Geometry: final body of the model. Coordinates: model frame, mm. A direction names the side the tool comes from. Round coordinates to 2 decimals unless told otherwise and drop trailing zeros. Loops run counter-clockwise (first coordinate to the right, second up) from the corner with the lowest first, then second, coordinate; pieces in that order, holes last. Notation, with made-up numbers: (-20.75, -33.75) - (-9.75, -33.75) arc R25 ccw to (-9.75, -10.75) - close; hole circle Ø5 at (58.5, -36.5). An arc over 180 degrees is marked (long way). Answer as a JSON object with one key per item and string values. Group by question number.
Item 1: Section A-A (y = -12). Return the cut outline in (x, z).
Item 2: Reachability of faces 5 (the face through (12.7, 122.6, -0.7)), 6 (the face through (15, -19.577, -11)), 7 (the face through (9, 45, 4.362)), 8 (the face through (2.58, -37.76, -9.25)) from +Z, -Z, +X, -X, +Y, -Y: full face, straight path, thin tool, end or side. Return the list, or none.
Item 3: Section D-D (y = 53). Return the cut outline in (x, z).
Item 4: Line query: line 1 (X direction, y = -14.5, z = -4.75); line 2 (Z direction, x = 2.75, y = 59); line 3 (Y direction, x = 10.25, z = -0.25). Output: solid intervals per line, ascending.
Item 5: Section C-C (x = 7.5). Return the cut outline in (y, z).
Item 6: Section B-B (x = 1.5). Return the cut outline in (y, z), plus the area to 3 significant figures.
Item 7: Draft query along Z for faces 1 (the face through (15, -28, -14.688)), 2 (the face through (3, -34, -8.338)), 3 (the face through (15.28, -37.76, -9.25)), 4 (the face through (0, 45, -3)). Return one class per face: released by +Z, released by -Z, zero draft, split by the parting line, or undercut.
Item 8: First-contact query: pin 1 (1.5 mm diameter, centred on x = 16.5, z = -13, fed in from +Y); pin 2 (3 mm diameter, centred on x = 10.5, z = -3, fed in from -Y); pin 3 (5 mm diameter, centred on x = 11, z = -4, fed in from -Y); pin 4 (4 mm diameter, centred on y = -32.28, z = -1.99, fed in from +X). Flat tips, straight axial feed; report the tip coordinate or a pass-through.
```python
from build123d import *

# Parameters (mm, degrees)
F0_W      = 63.5
F0_H      = 12.7
F1_DEPTH  = 17.78
F2_W      = 5.08
F2_H      = 12.7
F3_DEPTH  = 25.4
F4_R      = 2.54
F5_DEPTH  = 25.4
F6_DEPTH  = 50.8
F7_DEPTH  = 76.2
F8_W      = 5.08
F8_H      = 12.7
F9_DEPTH  = 12.7
F11_W     = 5.08
F11_H     = 12.7
F12_DEPTH = 6.35
F13_DEPTH = 6.35
F15_DEPTH = 25.4
F10_R     = 2.54
F16_DEPTH = 25.4
F14_R     = 1.2823476499
F17_DEPTH = 25.4


# Not quite as in the source:
# - a feature names something its author has since deleted; it is built from what else it names


with BuildPart() as f1:
    # F0 (on Right) → F1 (new body)
    with BuildSketch(Plane.YZ):
        with Locations((10.0746992975, -1.9877629941)):
            Rectangle(F0_W, F0_H)
    extrude(amount=F1_DEPTH)

    # F2 (on face) → F3 (join)
    with BuildSketch(Plane.XZ.offset(21.6753007025)):
        with Locations((2.54, -1.9877629941)):
            Rectangle(F2_W, F2_H)
        with Locations((15.24, -1.9877629941)):
            Rectangle(F2_W, F2_H)
    extrude(amount=F3_DEPTH)

    # F4 (on face) → F5 (cut)
    with BuildSketch(Plane.YZ.offset(17.78)):
        with Locations((-32.2765819728, -1.9877629941)):
            Circle(F4_R)
        with BuildLine():
            ThreePointArc((-32.2765819728, -8.3377629941), (-38.3512132445, -1.9877629941), (-32.2765819728, 4.3622370059))
            Line((-32.2765819728, 4.3622370059), (-47.0753007025, 4.3622370059))
            Line((-47.0753007025, 4.3622370059), (-47.0753007025, -8.3377629941))
            Line((-47.0753007025, -8.3377629941), (-32.2765819728, -8.3377629941))
        make_face()
    extrude(amount=-F5_DEPTH, mode=Mode.SUBTRACT)

    # F6 (cut): a face of the model
    f6_faces = [f1.faces().sort_by_distance(p)[0] for p in [
        (8.89, -21.6753007025, -1.9877629941),
    ]]
    extrude(f6_faces, amount=-F6_DEPTH, mode=Mode.SUBTRACT)

    # F7 (add): a face of the model
    f7_faces = [f1.faces().sort_by_distance(p)[0] for p in [
        (8.89, 41.8246992975, -1.9877629941),
    ]]
    extrude(f7_faces, amount=F7_DEPTH)

    # F8 (on face) → F9 (join)
    with BuildSketch(Plane(origin=(0, 118.0246992975, 0), x_dir=(-1, 0, 0), z_dir=(0, 1, 0))):
        with Locations((-15.24, -1.9877629941)):
            Rectangle(F8_W, F8_H)
        with Locations((-2.54, -1.9877629941)):
            Rectangle(F8_W, F8_H)
    extrude(amount=F9_DEPTH)

    # F11 (on face) → F12 (join)
    with BuildSketch(Plane(origin=(0, 0, -8.3377629941), x_dir=(1, 0, 0), z_dir=(0, 0, -1))):
        with Locations((15.24, 25.9265819728)):
            Rectangle(F11_W, F11_H)
        with Locations((2.54, 25.9265819728)):
            Rectangle(F11_W, F11_H)
    extrude(amount=F12_DEPTH)

    # F13 (add): faces of the model
    f13_faces = [f1.faces().sort_by_distance(p)[0] for p in [
        (15.24, -32.2765819728, -11.5127629941),
        (2.54, -32.2765819728, -11.5127629941),
    ]]
    extrude(f13_faces, amount=F13_DEPTH)

    # F14 (on face) → F15 (cut)
    with BuildSketch(Plane.YZ.offset(17.78)):
        with BuildLine():
            ThreePointArc((-38.6265819728, -10.9001689166), (-37.7400292742, -9.2277758835), (-36.0694751143, -8.3377629941))
            Line((-36.0694751143, -8.3377629941), (-38.6265819728, -8.3377629941))
            Line((-38.6265819728, -8.3377629941), (-38.6265819728, -10.9001689166))
        make_face()
        with BuildLine():
            ThreePointArc((-36.0694751143, -14.6877629941), (-37.7400292742, -13.7977501047), (-38.6265819728, -12.1253570717))
            Line((-38.6265819728, -12.1253570717), (-38.6265819728, -14.6877629941))
            Line((-38.6265819728, -14.6877629941), (-36.0694751143, -14.6877629941))
        make_face()
    extrude(amount=-F15_DEPTH, mode=Mode.SUBTRACT)

    # F10 (on face) → F16 (cut)
    with BuildSketch(Plane.YZ.offset(17.78)):
        with BuildLine():
            ThreePointArc((125.2040266991, 4.3622370059), (130.0066745518, -1.9877629941), (125.2040266991, -8.3377629941))
            Line((125.2040266991, -8.3377629941), (130.7246992975, -8.3377629941))
            Line((130.7246992975, -8.3377629941), (130.7246992975, 4.3622370059))
            Line((130.7246992975, 4.3622370059), (125.2040266991, 4.3622370059))
        make_face()
        with Locations((125.2040266991, -1.9877629941)):
            Circle(F10_R)
    extrude(amount=-F16_DEPTH, mode=Mode.SUBTRACT)

    # F14 (on face) → F17 (cut)
    with BuildSketch(Plane.YZ.offset(17.78)):
        with Locations((-36.0694751144, -11.5127629941)):
            Circle(F14_R)
    extrude(amount=-F17_DEPTH, mode=Mode.SUBTRACT)


solid = f1.part
```
Values:
{
 "1": {"outline": "(0, -8.34) - (5.08, -8.34) - (5.08, 4.36) - (0, 4.36) - close; (12.7, -8.34) - (17.78, -8.34) - (17.78, 4.36) - (12.7, 4.36) - close"},
 "2": {"face 5": "+Z, -Z, +Y", "face 6": "-Z, +X, -X, +Y", "face 7": "+Z, +X, -X, +Y, -Y", "face 8": "+X, -X, -Y"},
 "3": {"outline": "(0, -8.34) - (17.78, -8.34) - (17.78, 4.36) - (0, 4.36) - close"},
 "4": {"line 1": "x = 0 to 5.08, 12.7 to 17.78", "line 2": "z = -8.34 to 4.36", "line 3": "y = 29.12 to 118.02"},
 "5": {"outline": "(29.12, -8.34) - (118.02, -8.34) - (118.02, 4.36) - (29.12, 4.36) - close"},
 "6": {"outline": "(-38.63, -12.13) arc R3.23 ccw to (-36.07, -14.69) - (-19.58, -14.69) - (-19.58, -8.34) - (125.2, -8.34) arc R6.6 ccw to (125.2, 4.36) - (-32.28, 4.36) arc R6.36 ccw to (-32.28, -8.34) - (-36.07, -8.34) arc R3.23 ccw to (-38.63, -10.9) - close; hole circle Ø2.56 at (-36.07, -11.51); hole circle Ø5.08 at (-32.28, -1.99); hole circle Ø5.08 at (125.2, -1.99)", "area": "2,180 mm^2"},
 "7": {"face 1": "released by -Z", "face 2": "undercut", "face 3": "undercut", "face 4": "zero draft"},
 "8": {"pin 1": "stops at y = -19.58", "pin 2": "stops at y = 29.12", "pin 3": "stops at y = -38.35", "pin 4": "passes through"}
}
